```python
from build123d import *

# Parameters (mm, degrees)
DODANIE_WYCI_GNI_CIE1_DEPTH    = 100
WYTNIJ_WYCI_GNI_CIE1_DEPTH     = 5
OTW_R_GWINTOWANY_1_4_201_D     = 5.1054
OTW_R_GWINTOWANY_1_4_201_DEPTH = 8.64
OTW_R_GWINTOWANY_1_4_201_TIP   = 1.533816902


with BuildPart() as part:
    # Szkic1 → Dodanie-wyci_gni_cie1 (new body)
    with BuildSketch(Plane.XY):
        with BuildLine():
            Line((27.92734735, 15), (28.389677427, 14.733588619))
            ThreePointArc((28.389677427, 14.733588619), (30, 5), (31.610322573, 14.733588619))
            Line((31.610322573, 14.733588619), (32.07265265, 15))
            Line((32.07265265, 15), (35, 15))
            Line((35, 15), (40, 10))
            Line((40, 10), (40, 1))
            Line((40, 1), (39, 0))
            Line((39, 0), (-39, 0))
            Line((-39, 0), (-40, 1))
            Line((-40, 1), (-40, 10))
            Line((-40, 10), (-35, 15))
            Line((-35, 15), (-32.07265265, 15))
            Line((-32.07265265, 15), (-31.610322573, 14.733588619))
            ThreePointArc((-31.610322573, 14.733588619), (-30, 5), (-28.389677427, 14.733588619))
            Line((-28.389677427, 14.733588619), (-27.92734735, 15))
            Line((-27.92734735, 15), (27.92734735, 15))
        make_face()
    extrude(amount=DODANIE_WYCI_GNI_CIE1_DEPTH)

    # Szkic2 → Wytnij-wyci_gni_cie1 (cut)
    with BuildSketch(Plane(origin=(0, 0, 0), x_dir=(-1, 0, 0), z_dir=(0, -1, 0))):
        with BuildLine():
            ThreePointArc((2.408314264, -54.073430305), (2.279954566, -53.41770522), (2.593210084, -52.827516622))
            ThreePointArc((2.593210084, -52.827516622), (3.835217741, -49.896589795), (2.437074489, -47.036850202))
            ThreePointArc((2.437074489, -47.036850202), (2.086974186, -46.435257956), (2.214243, -45.750943625))
            Line((2.214243, -45.750943625), (26.605129776, -5))
            Line((26.605129776, -5), (26.605129776, -95))
            Line((26.605129776, -95), (4.967404335, -58.401883282))
            Line((4.967404335, -58.401883282), (2.408314264, -54.073430305))
        make_face()
        with BuildLine():
            Line((-24.302635093, -95), (24.281729572, -95))
            Line((24.281729572, -95), (0.200251555, -54.268512505))
            ThreePointArc((0.200251555, -54.268512505), (0.109677176, -54.139680814), (0, -54.02666648))
            ThreePointArc((0, -54.02666648), (-0.109677176, -54.139680814), (-0.200251555, -54.268512505))
            Line((-0.200251555, -54.268512505), (-24.302635093, -95))
        make_face()
        with BuildLine():
            ThreePointArc((-2.214243, -45.750943625), (-2.086974186, -46.435257956), (-2.437074489, -47.036850202))
            ThreePointArc((-2.437074489, -47.036850202), (-3.836608728, -50.004717824), (-2.429779642, -52.9691345))
            ThreePointArc((-2.429779642, -52.9691345), (-2.077967373, -53.571197168), (-2.205174034, -54.256813529))
            Line((-2.205174034, -54.256813529), (-26.605129776, -95))
            Line((-26.605129776, -95), (-26.605129776, -5))
            Line((-26.605129776, -5), (-2.214243, -45.750943625))
        make_face()
        with BuildLine():
            Line((-24.299393508, -5), (-0.317489033, -45.533191657))
            ThreePointArc((-0.317489033, -45.533191657), (-0.177941432, -45.716925413), (0, -45.863787501))
            ThreePointArc((0, -45.863787501), (0.177941432, -45.716925413), (0.317489033, -45.533191657))
            Line((0.317489033, -45.533191657), (24.281729572, -5))
            Line((24.281729572, -5), (-24.299393508, -5))
        make_face()
    extrude(amount=-WYTNIJ_WYCI_GNI_CIE1_DEPTH, mode=Mode.SUBTRACT)

    # Otw_r gwintowany 1_4-201
    with Locations(Plane(origin=(0, 0, 50), x_dir=(0, 0, -1), z_dir=(0, -1, 0))):
        with Locations((0, 0)):
            Hole(OTW_R_GWINTOWANY_1_4_201_D / 2, depth=OTW_R_GWINTOWANY_1_4_201_DEPTH)
            with Locations((0, 0, -(OTW_R_GWINTOWANY_1_4_201_DEPTH + OTW_R_GWINTOWANY_1_4_201_TIP / 2))):  # 118° drill point
                Cone(0, OTW_R_GWINTOWANY_1_4_201_D / 2, OTW_R_GWINTOWANY_1_4_201_TIP, mode=Mode.SUBTRACT)


solid = part.part
```
Geometry check sheet. Reference: the model listing, model coordinates, mm. A direction names the side the tool comes from. Coordinates: 2 decimals unless noted, no trailing zeros. Write each loop counter-clockwise with the first axis right and the second up, starting at its lowest first coordinate (ties: lowest second). Pieces come first, ordered by that corner, then holes. Notation, with made-up numbers: M 84.25,39 L 134.25,39 A13 cw 134.25,54 Z; hole C -29,-27 d6. An arc over 180 degrees is marked long. Answer as a JSON object with one key per item and string values.
1. Tool access check on faces 1 (the cylindrical face through (0.767, 4.38, 52.435)), 2 (the flat face through (0, 15, 49)). Record the directions out of +Z, -Z, +X, -X, +Y, -Y that give a thin tool (end or side, any length) a straight path to the whole face; none if there is none.
Answers below:
{"face 1": "-Y", "face 2": "+Z, -Z, +X, -X, +Y"}
2. Go/stop test with flat-tipped pins: pin 1 Ø2 at (x, z) = (11.5, 74) entering from -Y; pin 2 Ø6 at (x, y) = (30, 10) entering from +Z. Record where each tip stops, or that it passes through.
Answers below:
{"pin 1": "stops at y = 0", "pin 2": "passes through"}
3. Section check A-A, the plane y = 2.5. Enter the section's corners in (x, z), plus the area to 3 significant figures.
Answers below:
{"outline": "M -40,0 L 40,0 L 40,100 L -40,100 Z; hole M -26.61,5 L -2.21,45.75 A1 ccw -2.44,47.04 A3.84 cw -2.59,52.83 A1 ccw -2.41,54.07 L -26.61,95 Z; hole M -24.28,5 L 24.3,5 L 0.32,45.53 A1 ccw 0,45.86 A1 ccw -0.32,45.53 Z; hole M -24.28,95 L -0.2,54.27 A1 ccw 0,54.03 A1 ccw 0.2,54.27 L 24.3,95 Z; hole C 0,50 d5.11; hole M 2.21,45.75 L 26.61,5 L 26.61,95 L 2.21,54.26 A1 ccw 2.43,52.97 A3.84 cw 2.44,47.04 A1 ccw Z", "area": "3,600 mm²"}
4. Scan lines: L1, parallel to X at y = 10, z = 22; L2, parallel to Z at x = 0, y = 6.5; L3, parallel to X at y = 7.75, z = 24. Record each from-to range of solid material in increasing order.
Answers below:
{"L1": "x = -40 to -35, -25 to 25, 35 to 40", "L2": "z = 0 to 47.45, 52.55 to 100", "L3": "x = -40 to -34.47, -25.53 to 25.53, 34.47 to 40"}
5. Section check B-B, the plane z = 63. Enter the section's corners in (x, y).
Answers below:
{"outline": "M -40,1 L -39,0 L -26.61,0 L -26.61,5 L -7.69,5 L -7.69,0 L -5.36,0 L -5.36,5 L 5.37,5 L 5.37,0 L 7.44,0 L 7.44,5 L 26.61,5 L 26.61,0 L 39,0 L 40,1 L 40,10 L 35,15 L 32.07,15 L 31.61,14.73 A5 cw long 28.39,14.73 L 27.93,15 L -27.93,15 L -28.39,14.73 A5 cw long -31.61,14.73 L -32.07,15 L -35,15 L -40,10 Z"}
6. Section check D-D, the plane x = 19.5. Enter the section's corners in (y, z), plus the area to 3 significant figures.
Answers below:
{"outline": "M 0,0 L 15,0 L 15,100 L 0,100 L 0,95 L 5,95 L 5,86.88 L 0,86.88 L 0,83.14 L 5,83.14 L 5,16.87 L 0,16.87 L 0,13.11 L 5,13.11 L 5,5 L 0,5 Z", "area": "1,090 mm²"}
7. Section check C-C, the plane y = 11.75. Enter the section's corners in (x, z).
Answers below:
{"outline": "M -38.25,0 L -34.68,0 L -34.68,100 L -38.25,100 Z; M -25.32,0 L 25.32,0 L 25.32,100 L -25.32,100 Z; M 34.68,0 L 38.25,0 L 38.25,100 L 34.68,100 Z"}
8. Draft check along X on faces 3 (the flat face through (12.083, 2.465, 74.349)), 4 (the flat face through (40, 6, 49)), 5 (the flat face through (-38, 12, 49)). Enter one of: released by +X, released by -X, zero draft, split by the parting line, or undercut.
Answers below:
{"face 3": "undercut", "face 4": "released by +X", "face 5": "released by -X"}
